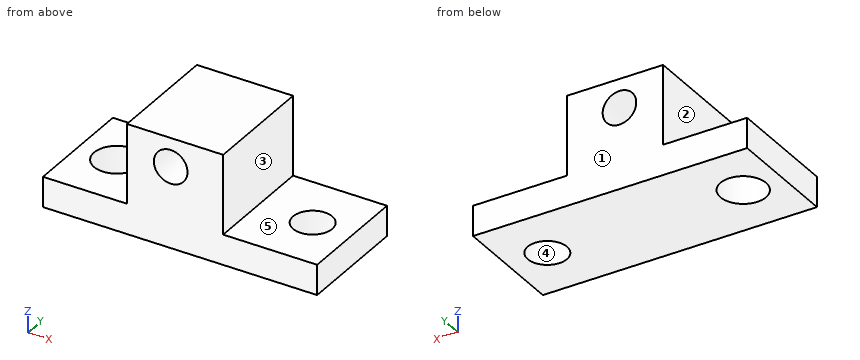
```python
from build123d import *

# Parameters (mm, degrees)
F0_R     = 10.025371
F1_DEPTH = 33.782
F2_DEPTH = 25.4
F3_R     = 13.556972
F3_R_2   = 11.687206
F4_DEPTH = 25.4
F5_DEPTH = 25.4


with BuildPart() as f1:
    # F0 (on Front) → F1 (new body, symmetric)
    with BuildSketch(Plane.XZ):
        Polygon((-76.107018, 18.011289), (-76.107018, 0), (87.307796, 0), (87.307796, 18.011289), (31.29869, 18.011289), (31.29869, 65.454304), (-26.03207, 65.454304), (-26.03207, 18.011289), align=None)
        with Locations((0, 48.306234)):
            Circle(F0_R, mode=Mode.SUBTRACT)
    extrude(amount=F1_DEPTH, both=True)

    # F0 (on Front) → F2 (join)
    with BuildSketch(Plane.XZ):
        Polygon((-76.107018, 18.011289), (-76.107018, 0), (87.307796, 0), (87.307796, 18.011289), (31.29869, 18.011289), (31.29869, 65.454304), (-26.03207, 65.454304), (-26.03207, 18.011289), align=None)
        with Locations((0, 48.306234)):
            Circle(F0_R, mode=Mode.SUBTRACT)
    extrude(amount=F2_DEPTH)

    # F3 (on face) → F4 (cut)
    with BuildSketch(Plane.XY.offset(18.011289)):
        with Locations((-52.955225, 0)):
            Circle(F3_R)
        with Locations((63.819543, 0)):
            Circle(F3_R_2)
    extrude(amount=-F4_DEPTH, mode=Mode.SUBTRACT)

    # F3 (on face) → F5 (cut)
    with BuildSketch(Plane.XY.offset(18.011289)):
        with Locations((-52.955225, 0)):
            Circle(F3_R)
        with Locations((63.819543, 0)):
            Circle(F3_R_2)
    extrude(amount=-F5_DEPTH, mode=Mode.SUBTRACT)


solid = f1.part
```
Geometry check sheet. Reference: the model listing, model coordinates, mm. Face numbers are marked on the shaded views. A direction names the side the tool comes from. Give positions to 0.01 mm unless a question says otherwise; leave off trailing zeros. Order: outer loops, then holes, each group sorted by start corner. A loop starts at its lowest first (then second) coordinate and runs counter-clockwise, first axis right, second up. Notation, with made-up numbers: (-5, 45.5) - (41, 45.5) arc R25 ccw to (41, 80.5) - close; hole circle Ø5 at (21.5, -31.75). An arc over 180 degrees is marked (long way). Write item = value, one per line. Start each with the question number.
1) Section check C-C (z = 9). Enter the section's corners in (x, y), then the cut area to 3 significant figures.
2) Access from +Z, -Z, +X, -X, +Y, -Y to the whole of each face (thin tool, end or side, straight path). Record for the marked faces 1 and 2.
3) Draft check along X on the marked faces 3, 4 and 5. Enter one of: released by +X, released by -X, zero draft, split by the parting line, or undercut.
4) Section check A-A (y = 0). Enter the section's corners in (x, z).
5) Section check D-D (y = 25.5). Enter the section's corners in (x, z).
6) Gauge pin test, flat ends, axial feed: pin 1 Ø14 at (y, z) = (7.5, 33) entering from +X; pin 2 Ø15 at (x, y) = (-46.5, 8) entering from +Z; pin 3 Ø14 at (y, z) = (3.5, 34.5) entering from -X. Record the tip position at first contact, or that the pin passes through.
7) Scan lines: L1, parallel to X at y = 29.5, z = 48; L2, parallel to Z at x = 0, y = 20; L3, parallel to Z at x = -44, y = -15. Record each from-to range of solid material in increasing order.
8) Section check B-B (x = 0). Enter the section's corners in (y, z), then the cut area to 3 significant figures.
Geometry check:
q1.outline = (-76.11, -33.78) - (87.31, -33.78) - (87.31, 33.78) - (-76.11, 33.78) - close; hole circle Ø27.11 at (-52.96, 0); hole circle Ø23.37 at (63.82, 0)
q1.area = 10,000 mm2
q2.face_1 = +Z, -Z, +X, -X, +Y
q2.face_2 = +Z, -X, +Y, -Y
q3.face_3 = released by +X
q3.face_4 = undercut
q3.face_5 = zero draft
q4.outline = (-76.11, 0) - (-66.51, 0) - (-66.51, 18.01) - (-76.11, 18.01) - close; (-39.4, 0) - (52.13, 0) - (52.13, 18.01) - (31.3, 18.01) - (31.3, 65.45) - (-26.03, 65.45) - (-26.03, 18.01) - (-39.4, 18.01) - close; (75.51, 0) - (87.31, 0) - (87.31, 18.01) - (75.51, 18.01) - close; hole circle Ø20.05 at (0, 48.31)
q5.outline = (-76.11, 0) - (87.31, 0) - (87.31, 18.01) - (31.3, 18.01) - (31.3, 65.45) - (-26.03, 65.45) - (-26.03, 18.01) - (-76.11, 18.01) - close; hole circle Ø20.05 at (0, 48.31)
q6.pin_1 = 31.3
q6.pin_2 = 18.01
q6.pin_3 = -26.03
q7.L1 = -26.03 to -10.02, 10.02 to 31.3
q7.L2 = 0 to 38.28, 58.33 to 65.45
q7.L3 = 0 to 18.01
q8.outline = (-33.78, 0) - (33.78, 0) - (33.78, 38.28) - (-33.78, 38.28) - close; (-33.78, 58.33) - (33.78, 58.33) - (33.78, 65.45) - (-33.78, 65.45) - close
q8.area = 3,070 mm2
